```python
from build123d import *

# Parameters (mm, degrees)
SKETCH1_W            = 27
SKETCH1_H            = 27
SKETCH1_W_2          = 23
SKETCH1_H_2          = 23
BOSS_EXTRUDE1_DEPTH  = 2
SKETCH2_W            = 27
SKETCH2_H            = 27
BOSS_EXTRUDE2_DEPTH  = 2
SKETCH12_W           = 5
SKETCH12_H           = 4
BOSS_EXTRUDE9_DEPTH  = 6
SKETCH13_R           = 1.75
CUT_EXTRUDE4_DEPTH   = 2
LPATTERN3_COUNT      = 6
LPATTERN3_PITCH      = 3.75
LPATTERN3_COUNT_DIR2 = 6
LPATTERN3_PITCH_DIR2 = 3.75
CUT_EXTRUDE5_REACH   = 18
SKETCH14_W           = 27
SKETCH14_H           = 27
SKETCH14_W_2         = 23
SKETCH14_H_2         = 23
BOSS_EXTRUDE10_DEPTH = 8.5
BOSS_EXTRUDE11_DEPTH = 23
SKETCH18_W           = 27
SKETCH18_H           = 27
BOSS_EXTRUDE12_DEPTH = 2
SKETCH17_R           = 4.25
CUT_EXTRUDE10_DEPTH  = 2
SKETCH19_R           = 0.5
BOSS_EXTRUDE13_DEPTH = 6.51087


with BuildPart() as part:
    # Sketch1 → Boss-Extrude1 (new body)
    with BuildSketch(Plane(origin=(0, 0, 0), x_dir=(1, 0, 0), z_dir=(0, 1, 0))):
        Rectangle(SKETCH1_W, SKETCH1_H)
        Rectangle(SKETCH1_W_2, SKETCH1_H_2, mode=Mode.SUBTRACT)
    extrude(amount=BOSS_EXTRUDE1_DEPTH)

    # Sketch2 → Boss-Extrude2 (add)
    with BuildSketch(Plane.XZ):
        Rectangle(SKETCH2_W, SKETCH2_H)
    extrude(amount=BOSS_EXTRUDE2_DEPTH)

    # Sketch12 → Boss-Extrude9 (add)
    with BuildSketch(Plane.ZY.offset(13.5)):
        Rectangle(SKETCH12_W, SKETCH12_H)
    boss_extrude9 = extrude(amount=BOSS_EXTRUDE9_DEPTH)

    # Mirror1: Boss-Extrude9 across plane
    add(boss_extrude9.mirror(Plane(origin=(0, 0, 0), x_dir=(0, 0, 1), z_dir=(1, 0, 0))))

    # Sketch13 → Cut-Extrude4 (cut)
    with BuildSketch(Plane(origin=(0, 0, 0), x_dir=(1, 0, 0), z_dir=(0, 1, 0))):
        with Locations((9.5, 9.5)):
            Circle(SKETCH13_R)
    cut_extrude4 = extrude(amount=-CUT_EXTRUDE4_DEPTH, mode=Mode.SUBTRACT)

    # LPattern3: Cut-Extrude4 6 × 6
    with Locations(*[(-j * LPATTERN3_PITCH_DIR2, 0, i * LPATTERN3_PITCH) for i in range(LPATTERN3_COUNT) for j in range(LPATTERN3_COUNT_DIR2) if (i, j) != (0, 0)]):
        add(cut_extrude4, mode=Mode.SUBTRACT)

    # Sketch15 → Cut-Extrude5 (cut, up to next)
    with BuildSketch(Plane.XY.offset(2.5), mode=Mode.PRIVATE) as cut_extrude5_sk1:
        with BuildLine():
            Line((-17.5, -2), (-15.5, -2))
            ThreePointArc((-15.5, -2), (-16.5, -1), (-17.5, -2))
        make_face()
    cut_extrude5_tool1 = extrude(cut_extrude5_sk1.sketch, amount=-CUT_EXTRUDE5_REACH, mode=Mode.PRIVATE) & part.part
    add(cut_extrude5_tool1.solids().sort_by_distance((-16.5, -1.575587, 2.5))[0], mode=Mode.SUBTRACT)
    # Sketch15 → Cut-Extrude5 (cut, up to next)
    with BuildSketch(Plane.XY.offset(2.5), mode=Mode.PRIVATE) as cut_extrude5_sk2:
        with BuildLine():
            Line((17.5, -2), (15.5, -2))
            ThreePointArc((15.5, -2), (16.5, -1), (17.5, -2))
        make_face()
    cut_extrude5_tool2 = extrude(cut_extrude5_sk2.sketch, amount=-CUT_EXTRUDE5_REACH, mode=Mode.PRIVATE) & part.part
    add(cut_extrude5_tool2.solids().sort_by_distance((16.5, -1.575587, 2.5))[0], mode=Mode.SUBTRACT)

    # Sketch14 → Boss-Extrude10 (add)
    with BuildSketch(Plane.XZ.offset(2)):
        Rectangle(SKETCH14_W, SKETCH14_H)
        Rectangle(SKETCH14_W_2, SKETCH14_H_2, mode=Mode.SUBTRACT)
    extrude(amount=BOSS_EXTRUDE10_DEPTH)

    # Sketch16 → Boss-Extrude11 (add)
    with BuildSketch(Plane.ZY.offset(-11.5)):
        Polygon((11.5, -10.5), (-11.5, -10.5), (-11.5, -9.5), (11.5, -3), align=None)
    extrude(amount=BOSS_EXTRUDE11_DEPTH)

    # Sketch18 → Boss-Extrude12 (add)
    with BuildSketch(Plane.XZ.offset(10.5)):
        Rectangle(SKETCH18_W, SKETCH18_H)
    extrude(amount=BOSS_EXTRUDE12_DEPTH)

    # Sketch17 → Cut-Extrude10 (cut)
    with BuildSketch(Plane(origin=(0, 0, -13.5), x_dir=(-1, 0, 0), z_dir=(0, 0, -1))):
        with Locations((0, -6.25)):
            Circle(SKETCH17_R)
    extrude(amount=-CUT_EXTRUDE10_DEPTH, mode=Mode.SUBTRACT)

    # Sketch19 → Boss-Extrude13 (add)
    with BuildSketch(Plane.XZ.offset(2)):
        Circle(SKETCH19_R)
        with Locations((3.75, 0)):
            Circle(SKETCH19_R)
        with Locations((0, 3.75)):
            Circle(SKETCH19_R)
        with Locations((-3.75, 3.75)):
            Circle(SKETCH19_R)
        with Locations((3.75, 3.75)):
            Circle(SKETCH19_R)
        with Locations((7.5, 3.75)):
            Circle(SKETCH19_R)
        with Locations((7.5, 7.5)):
            Circle(SKETCH19_R)
        with Locations((3.75, 7.5)):
            Circle(SKETCH19_R)
        with Locations((0, 7.5)):
            Circle(SKETCH19_R)
        with Locations((-3.75, 7.5)):
            Circle(SKETCH19_R)
        with Locations((-7.5, 7.5)):
            Circle(SKETCH19_R)
        with Locations((-7.5, 3.75)):
            Circle(SKETCH19_R)
        with Locations((-7.5, 0)):
            Circle(SKETCH19_R)
        with Locations((-3.75, 0)):
            Circle(SKETCH19_R)
        with Locations((-3.75, -3.75)):
            Circle(SKETCH19_R)
        with Locations((-7.5, -3.75)):
            Circle(SKETCH19_R)
        with Locations((-7.5, -7.5)):
            Circle(SKETCH19_R)
        with Locations((-3.75, -7.5)):
            Circle(SKETCH19_R)
        with Locations((0, -7.5)):
            Circle(SKETCH19_R)
        with Locations((0, -3.75)):
            Circle(SKETCH19_R)
        with Locations((3.75, -3.75)):
            Circle(SKETCH19_R)
        with Locations((3.75, -7.5)):
            Circle(SKETCH19_R)
        with Locations((7.5, -7.5)):
            Circle(SKETCH19_R)
        with Locations((7.5, -3.75)):
            Circle(SKETCH19_R)
        with Locations((7.5, 0)):
            Circle(SKETCH19_R)
    extrude(amount=BOSS_EXTRUDE13_DEPTH)


solid = part.part
```
Here's how the part is built. I have some questions about the finished solid (model axes, mm). A direction names the side the tool comes from. Round coordinates to 2 decimals unless told otherwise and drop trailing zeros. Order: outer loops, then holes, each group sorted by start corner. A loop starts at its lowest first (then second) coordinate and runs counter-clockwise, first axis right, second up. Notation, with made-up numbers: M 21.25,-38.75 L 50.25,-38.75 A7 ccw 50.25,-26.75 Z; hole C 2,-37 d9. An arc over 180 degrees is marked long. One line per question, with ' | ' between items.
1) I want a section at A-A, the plane z = -5.75. State how many separate pieces and enclosed holes the cut face has, then the cut area to 3 significant figures.
Working result:
separate pieces: 6 | enclosed holes: 0 | area: 168 mm²
2) For pin 1 Ø1.6 at (y, z) = (1, 4.5) entering from -X; pin 2 Ø3 at (x, z) = (5.75, -2) entering from +Y; pin 3 Ø1.2 at (x, y) = (15.5, -1) entering from +Z, each with a flat end and sliding along its axis, tell me the tip position at first contact or that it passes through.
Working result:
pin 1: x = -13.5 | pin 2: y = -6.39 | pin 3: z = 2.5
3) I want a section at C-C, the plane y = -11.5. Write out the boundary of the cut face in (x, z).
Working result:
outline: M -13.5,-13.5 L 13.5,-13.5 L 13.5,13.5 L -13.5,13.5 Z
4) I need wall thicknesses on line 1 along X through (y, z) = (1.25, -6.5); line 2 along Z through (x, y) = (17, 0); line 3 along X through (y, z) = (-0.5, 11.75). Which ranges of each line are inside material? Lowest first, please.
Working result:
line 1: -13.5 to -11.5, 11.5 to 13.5 | line 2: -2.5 to 2.5 | line 3: -13.5 to 13.5
5) If we mould it in two halves opening along Z, with no side actions, what happens to faces 1 (the face through (0, -12.5, 0)), 2 (the face through (0, -10, -11.5)), 3 (the face through (0, 1, -11.5))? For each: +Z half, -Z half, draft (parallel to the pull), parting line (faces both ways), or undercut.
Working result:
face 1: draft | face 2: -Z half | face 3: undercut
6) For faces 4 (the face through (0.553, -2.036, -12.514)), 5 (the face through (-0.108, -4.179, -0.488)), 6 (the face through (-0.133, -0.986, -1.33)), which set-ups out of +Z, -Z, +X, -X, +Y, -Y let a thin tool reach every point of the face, with its end or its side?
Working result:
face 4: -Z | face 5: none | face 6: +Y
